The model under review builds one solid part; all positions refer to its coordinate system, in mm. A direction names the side the tool comes from. Coordinates: 2 decimals unless noted, no trailing zeros. Write each loop counter-clockwise with the first axis right and the second up, starting at its lowest first coordinate (ties: lowest second). Pieces come first, ordered by that corner, then holes. Notation, with made-up numbers: (77, 89) - (132, 89) arc R19 cw to (132, 118) - close; hole circle Ø10 at (-12, -28). An arc over 180 degrees is marked (long way). Return JSON: item names as keys, results as strings. Group by question number.
(1) We need section C-C on y = -3.5. State the section outline as (x, z) points, then the cut area to 3 significant figures.
(2) We need section A-A on z = 7.25. State the section outline as (x, y) points.
(3) To check wall thickness, follow L1, parallel to Y at x = 0, z = 9.5; L2, parallel to Y at x = 0, z = 6.75; L3, parallel to Z at x = 7.25, y = -3.25. State the ranges of each line that lie inside material, in increasing order. Write a range as from..to.
(4) We need section D-D on z = 4. State the section outline as (x, y) points, then the cut area to 3 significant figures.
(5) We need section B-B on x = 1.75. State the section outline as (y, z) points, then the cut area to 3 significant figures.
(6) Tool access review of faces 1 (the face through (-4, -2, 8)), 2 (the face through (1, 1, 13)): name each direction out of +Z, -Z, +X, -X, +Y, -Y from which nothing blocks a thin tool from reaching the whole face with its end or side.
(7) Draft analysis for pull direction Y (two halves, no side actions). For faces 3 (the face through (0.27, -1.22, 8.69)), 4 (the face through (0, 0, 0)), 5 (the face through (-0.867, -3.905, 10.465)), state which applies: released by +Y, released by -Y, zero draft, split by the parting line, or undercut.
(8) For pin 1 Ø3 at (x, z) = (-4, 4.5) entering from +Y; pin 2 Ø1 at (x, y) = (-5.5, 5) entering from +Z; pin 3 Ø1 at (y, z) = (-4, 5.5) entering from +X, all flat-tipped, find the tip position at first contact; note any pin that passes through.
```python
from build123d import *

# Parameters (mm, degrees)
SKETCH1_R             = 8
BOSS_EXTRUDE1_DEPTH   = 8
SKETCH2_R             = 4
BOSS_EXTRUDE2_DEPTH   = 5
M3_TAPPED_HOLE1_D     = 2.5
M3_TAPPED_HOLE1_DEPTH = 8.5
M3_TAPPED_HOLE1_TIP   = 0.751075774


with BuildPart() as part:
    # Sketch1 → Boss-Extrude1 (new body)
    with BuildSketch(Plane.XY):
        Circle(SKETCH1_R)
    extrude(amount=BOSS_EXTRUDE1_DEPTH)

    # Sketch2 → Boss-Extrude2 (add)
    with BuildSketch(Plane.XY.offset(8)):
        Circle(SKETCH2_R)
    extrude(amount=BOSS_EXTRUDE2_DEPTH)

    # M3 Tapped Hole1
    with Locations(Plane.XY.offset(13)):
        with Locations((0, 0)):
            Hole(M3_TAPPED_HOLE1_D / 2, depth=M3_TAPPED_HOLE1_DEPTH)
            with Locations((0, 0, -(M3_TAPPED_HOLE1_DEPTH + M3_TAPPED_HOLE1_TIP / 2))):  # 118° drill point
                Cone(0, M3_TAPPED_HOLE1_D / 2, M3_TAPPED_HOLE1_TIP, mode=Mode.SUBTRACT)


solid = part.part
```
Ans:
{
 "1": {"outline": "(-7.19, 0) - (7.19, 0) - (7.19, 8) - (1.94, 8) - (1.94, 13) - (-1.94, 13) - (-1.94, 8) - (-7.19, 8) - close", "area": "134 mm²"},
 "2": {"outline": "circle Ø16 at (0, 0); hole circle Ø2.5 at (0, 0)"},
 "3": {"L1": "-4..-1.25, 1.25..4", "L2": "-8..-1.25, 1.25..8", "L3": "0..8"},
 "4": {"outline": "circle Ø16 at (0, 0); hole circle Ø0.84 at (0, 0)", "area": "201 mm²"},
 "5": {"outline": "(-7.81, 0) - (7.81, 0) - (7.81, 8) - (3.6, 8) - (3.6, 13) - (-3.6, 13) - (-3.6, 8) - (-7.81, 8) - close", "area": "161 mm²"},
 "6": {"face 1": "+Z", "face 2": "+Z, +X, -X, +Y, -Y"},
 "7": {"face 3": "undercut", "face 4": "zero draft", "face 5": "split by the parting line"},
 "8": {"pin 1": "y = 7.6", "pin 2": "z = 8", "pin 3": "x = 7.19"}
}
